Read the model definition and answer for the solid it produces. Units are mm, in the model's axes. Face numbers are marked on the shaded views. Give positions to 0.01 mm unless a question says otherwise; leave off trailing zeros. Order: outer loops, then holes, each group sorted by start corner. A loop starts at its lowest first (then second) coordinate and runs counter-clockwise, first axis right, second up. Notation, with made-up numbers: (-15.75, 66) - (-7.75, 66) arc R17 cw to (-7.75, 97) - close; hole circle Ø2 at (-32.75, 36.25). An arc over 180 degrees is marked (long way). Answer as CSV lines item,"result". Start each with the question number.
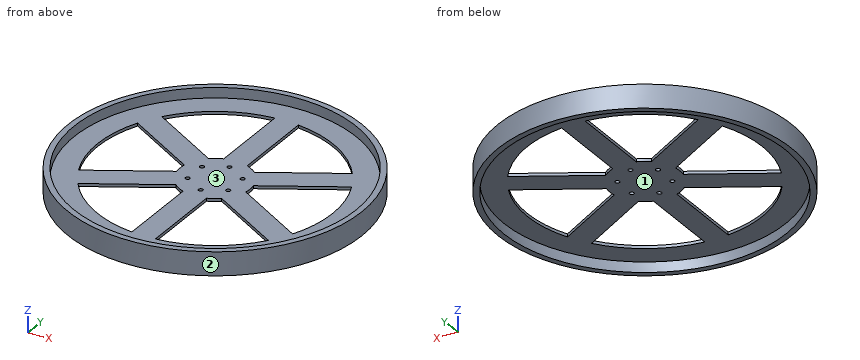
from build123d import *

# Parameters (mm, degrees)
SKETCH2_R                = 304.8
BOSS_EXTRUDE1_DEPTH      = 3.175
BOSS_EXTRUDE1_DEPTH_BACK = 3.175
SKETCH5_R                = 317.5
SKETCH5_R_2              = 304.8
BOSS_EXTRUDE2_DEPTH      = 25.4
BOSS_EXTRUDE2_DEPTH_BACK = 25.4
SKETCH6_R                = 4.7625
CUT_EXTRUDE4_DEPTH       = 29.575


with BuildPart() as part:
    # Sketch2 → Boss-Extrude1 (new body, two sides)
    with BuildSketch(Plane.XY) as boss_extrude1_sk:
        Circle(SKETCH2_R)
        with BuildLine():
            Line((25.4, -252.726809025), (25.4, -71.842048969))
            ThreePointArc((25.4, -71.842048969), (38.1, -65.991135768), (49.517039467, -57.91806974))
            Line((49.517039467, -57.91806974), (206.167836833, -148.360449769))
            ThreePointArc((206.167836833, -148.360449769), (127, -219.970452561), (25.4, -252.726809025))
        make_face(mode=Mode.SUBTRACT)
        with BuildLine():
            Line((231.567836833, -104.366359256), (74.917039467, -13.923979228))
            ThreePointArc((74.917039467, -13.923979228), (76.2, 0), (74.917039467, 13.923979228))
            Line((74.917039467, 13.923979228), (231.567836833, 104.366359256))
            ThreePointArc((231.567836833, 104.366359256), (254, 0), (231.567836833, -104.366359256))
        make_face(mode=Mode.SUBTRACT)
        with BuildLine():
            Line((206.167836833, 148.360449769), (49.517039467, 57.91806974))
            ThreePointArc((49.517039467, 57.91806974), (38.1, 65.991135768), (25.4, 71.842048969))
            Line((25.4, 71.842048969), (25.4, 252.726809025))
            ThreePointArc((25.4, 252.726809025), (127, 219.970452561), (206.167836833, 148.360449769))
        make_face(mode=Mode.SUBTRACT)
        with BuildLine():
            Line((-25.4, 252.726809025), (-25.4, 71.842048969))
            ThreePointArc((-25.4, 71.842048969), (-38.1, 65.991135768), (-49.517039467, 57.91806974))
            Line((-49.517039467, 57.91806974), (-206.167836833, 148.360449769))
            ThreePointArc((-206.167836833, 148.360449769), (-127, 219.970452561), (-25.4, 252.726809025))
        make_face(mode=Mode.SUBTRACT)
        with BuildLine():
            Line((-231.567836833, 104.366359256), (-74.917039467, 13.923979228))
            ThreePointArc((-74.917039467, 13.923979228), (-76.2, 0), (-74.917039467, -13.923979228))
            Line((-74.917039467, -13.923979228), (-231.567836833, -104.366359256))
            ThreePointArc((-231.567836833, -104.366359256), (-254, 0), (-231.567836833, 104.366359256))
        make_face(mode=Mode.SUBTRACT)
        with BuildLine():
            Line((-206.167836833, -148.360449769), (-49.517039467, -57.91806974))
            ThreePointArc((-49.517039467, -57.91806974), (-38.1, -65.991135768), (-25.4, -71.842048969))
            Line((-25.4, -71.842048969), (-25.4, -252.726809025))
            ThreePointArc((-25.4, -252.726809025), (-127, -219.970452561), (-206.167836833, -148.360449769))
        make_face(mode=Mode.SUBTRACT)
    extrude(amount=BOSS_EXTRUDE1_DEPTH)
    extrude(boss_extrude1_sk.sketch, amount=-BOSS_EXTRUDE1_DEPTH_BACK)

    # Sketch5 → Boss-Extrude2 (add, two sides)
    with BuildSketch(Plane.XY) as boss_extrude2_sk:
        Circle(SKETCH5_R)
        Circle(SKETCH5_R_2, mode=Mode.SUBTRACT)
    extrude(amount=BOSS_EXTRUDE2_DEPTH)
    extrude(boss_extrude2_sk.sketch, amount=-BOSS_EXTRUDE2_DEPTH_BACK)

    # Sketch6 → Cut-Extrude4 (cut, through all)
    with BuildSketch(Plane.XY.offset(3.175)):
        with Locations((0, 50.8)):
            Circle(SKETCH6_R)
        with Locations((43.994090512, 25.4)):
            Circle(SKETCH6_R)
        with Locations((43.994090512, -25.4)):
            Circle(SKETCH6_R)
        with Locations((0, -50.8)):
            Circle(SKETCH6_R)
        with Locations((-43.994090512, -25.4)):
            Circle(SKETCH6_R)
        with Locations((-43.994090512, 25.4)):
            Circle(SKETCH6_R)
    extrude(amount=-CUT_EXTRUDE4_DEPTH, mode=Mode.SUBTRACT)


solid = part.part
(1) Section A-A, the plane x = 195.5 is taken. Write down the section's boundary in (y, z) (3 decimals).
(2) Section C-C, the plane z = 15.5 is taken. Write down the section's boundary in (x, y).
(3) Straight lines are drawn through the part: line 1 (Y direction, x = 0, z = -1.5); line 2 (Y direction, x = 0, z = -18.75); line 3 (X direction, y = -62, z = 1). For each, find the intervals that lie inside material, in ascending order. Write a range as [from, to].
(4) Section D-D, the plane x = -103.5 is taken. Write down the section's boundary in (y, z) (3 decimals), and give its area (3 significant figures).
(5) Section B-B, the plane y = 217.5 is taken. Write down the section's boundary in (x, z) (3 decimals), and give its area (3 significant figures).
(6) Flat-ended cylindrical pins translate along their axes: pin 1 Ø8 at (y, z) = (47, -15) entering from +X; pin 2 Ø12.5 at (x, y) = (0, -50.8) entering from +Z (3 decimals); pin 3 Ø10 at (y, z) = (61.5, 8) entering from -X. Find the tip coordinate at first contact, or state that the pin passes through.
(7) Determine the mould class of the marked faces 1, 2 and 3 for opening direction X: released by +X, released by -X, zero draft, split by the parting line, or undercut.
Checks:
1,outline,"(-250.172, -25.4) - (-233.844, -25.4) - (-233.844, -3.175) - (-162.16, -3.175) - (-162.16, 3.175) - (-233.844, 3.175) - (-233.844, 25.4) - (-250.172, 25.4) - close; (-142.201, -3.175) - (-83.543, -3.175) - (-83.543, 3.175) - (-142.201, 3.175) - close; (83.543, -3.175) - (142.201, -3.175) - (142.201, 3.175) - (83.543, 3.175) - close; (162.16, -3.175) - (233.844, -3.175) - (233.844, -25.4) - (250.172, -25.4) - (250.172, 25.4) - (233.844, 25.4) - (233.844, 3.175) - (162.16, 3.175) - close"
2,outline,"circle Ø635 at (0, 0); hole circle Ø609.6 at (0, 0)"
3,line 1,"y = [-317.5, -55.56], [-46.04, 46.04], [55.56, 317.5]"
3,line 2,"y = [-317.5, -304.8], [304.8, 317.5]"
3,line 3,"x = [-311.39, -246.32], [-158.19, -56.59], [-44.3, 44.3], [56.59, 158.19], [246.32, 311.39]"
4,outline,"(-300.157, -25.4) - (-286.689, -25.4) - (-286.689, -3.175) - (-231.956, -3.175) - (-231.956, 3.175) - (-286.689, 3.175) - (-286.689, 25.4) - (-300.157, 25.4) - close; (-89.085, -3.175) - (-30.426, -3.175) - (-30.426, 3.175) - (-89.085, 3.175) - close; (30.426, -3.175) - (89.085, -3.175) - (89.085, 3.175) - (30.426, 3.175) - close; (231.956, -3.175) - (286.689, -3.175) - (286.689, -25.4) - (300.157, -25.4) - (300.157, 25.4) - (286.689, 25.4) - (286.689, 3.175) - (231.956, 3.175) - close"
4,area,"2,810 mm²"
5,outline,"(-231.301, -25.4) - (-213.534, -25.4) - (-213.534, -3.175) - (-131.186, -3.175) - (-131.186, 3.175) - (-213.534, 3.175) - (-213.534, 25.4) - (-231.301, 25.4) - close; (-25.4, -3.175) - (25.4, -3.175) - (25.4, 3.175) - (-25.4, 3.175) - close; (131.186, -3.175) - (213.534, -3.175) - (213.534, -25.4) - (231.301, -25.4) - (231.301, 25.4) - (213.534, 25.4) - (213.534, 3.175) - (131.186, 3.175) - close"
5,area,"3,170 mm²"
6,pin 1,"stops at x = 314.57"
6,pin 2,"stops at z = 3.175"
6,pin 3,"stops at x = -312.43"
7,face 1,"undercut"
7,face 2,"split by the parting line"
7,face 3,"undercut"
